Model file for the job. Use its own axes, mm. A direction names the side the tool comes from. Give positions to 0.01 mm unless a question says otherwise; leave off trailing zeros. Loops run counter-clockwise (first coordinate to the right, second up) from the corner with the lowest first, then second, coordinate; pieces in that order, holes last. Notation, with made-up numbers: M 49,34 L 54,34 A25 ccw 54,51 Z; hole C -3.5,14 d11. An arc over 180 degrees is marked long. Use CSV: the item, a comma, the result in double quotes. Start each with the question number.
(1) Flat gauge pins, fed straight in: P1, Ø1.1, axis at x = 0, y = -0.5, coming from the -Z side (3 decimals); P2, Ø0.8, axis at x = 0, z = -0.5, coming from the +Y side; P3, Ø1.4, axis at y = -1, z = 17.5, coming from the -X side (3 decimals). Where does each tip first touch, or does it go through?
(2) Tool access for faces 1 (the face through (0, -1.67, 17)), 2 (the face through (0, -1, -1.445)), 3 (the face through (0, -1, -1.245)), 4 (the face through (0, -1.47, 17)): list every direction of +Z, -Z, +X, -X, +Y, -Y with a clear straight run to the whole face (end or side of a thin tool).
(3) Wall check: line 1 along Z through (x, y) = (0, -1.4) (3 decimals); line 2 along Z through (x, y) = (0.35, -0.5) (3 decimals); line 3 along Y through (x, z) = (0.5, 12). Give the ranges that are in metal, low to high. Write a range as from..to.
(4) Slice it at A-A on y = -0.35. State how many separate pieces and enclosed holes the cut face has, and give its area (3 significant figures).
(5) Slice it at B-B on z = 10.25. List the corners of the cut face in (x, y).
```python
from build123d import *

# Parameters (mm, degrees)
SKETCH1_R        = 1.14
EXTRUSION1_DEPTH = 15.24
EXTRUSION2_DEPTH = 0.495
FILLET3_R        = 1.03


with BuildPart() as part:
    # Sketch1 → Extrusion1 (new body)
    with BuildSketch(Plane.XY):
        Circle(SKETCH1_R)
    extrude(amount=EXTRUSION1_DEPTH)

    # Sketch3 → Revolution3 (revolve, cut)
    with BuildSketch(Plane.YZ, mode=Mode.PRIVATE) as revolution3_sk:
        with BuildLine():
            Line((1.14, 12.96), (1.14, 14.1))
            ThreePointArc((1.14, 14.1), (1.101155442, 13.804946289), (0.98726896, 13.53))
            ThreePointArc((0.98726896, 13.53), (1.101155442, 13.255053711), (1.14, 12.96))
        make_face()
    revolution3 = revolve(revolution3_sk.sketch.rotate(Axis((0, 0, 14.1), (0, 0, -1)), 90), axis=Axis((0, 0, 14.1), (0, 0, -1)), mode=Mode.SUBTRACT)

    # Mirror2: Revolution3 across plane
    add(revolution3.mirror(Plane.XY.offset(7.62)), mode=Mode.SUBTRACT)

    # Sketch4 → Extrusion2 (add, symmetric)
    with BuildSketch(Plane.YZ):
        with BuildLine():
            Line((-0.1, 0), (0, 0))
            ThreePointArc((0, 0), (-0.050048254, 0.001099138), (-0.1, 0.004394435))
            Line((-0.1, 0.004394435), (-0.1, 0))
        make_face()
        with BuildLine():
            ThreePointArc((0, 0), (0.050048254, 0.001099138), (0.1, 0.004394435))
            Line((0.1, 0.004394435), (0.1, 0.138771336))
            Line((0.1, 0.138771336), (-0.1, 0.138771336))
            Line((-0.1, 0.138771336), (-0.1, 0.004394435))
            ThreePointArc((-0.1, 0.004394435), (-0.050048254, 0.001099138), (0, 0))
        make_face()
        Polygon((0.1, -1.445), (0.1, 0), (0, 0), (-0.1, 0), (-0.1, -1.245), (-1.67, -1.245), (-1.67, -2.925), (-1.47, -2.925), (-1.47, -1.445), align=None)
    extrusion2 = extrude(amount=EXTRUSION2_DEPTH, both=True)

    # Mirror3: Extrusion2 across plane
    add(extrusion2.mirror(Plane.XY.offset(7.62)))

    # Fillet3
    # the kernel refuses this fillet: 1.03 mm, written as the material it takes off along each edge
    with BuildSketch(Plane(origin=(0, 0, 15.24), x_dir=(1, 0, 0), z_dir=(0, -1, 0))) as fillet3_piece_1_section:
        with BuildLine():
            CenterArc((1.14 - FILLET3_R, -FILLET3_R), FILLET3_R, 0, 90)
            Line((1.14 - FILLET3_R, 0), (1.14, 0))
            Line((1.14, 0), (1.14, -FILLET3_R))
        make_face()
    fillet3_piece_1 = revolve(axis=Axis((0, 0, 15.24), (0, 0, 1)), mode=Mode.PRIVATE)
    fillet3_piece_1 = split(fillet3_piece_1, bisect_by=Plane(origin=(0.495, 4e-09, 15.000808078), z_dir=(1, 0, 0)), keep=Keep.TOP, mode=Mode.PRIVATE)
    add(fillet3_piece_1, mode=Mode.SUBTRACT)
    with BuildSketch(Plane(origin=(0, 0, 15.24), x_dir=(1, 0, 0), z_dir=(0, -1, 0))) as fillet3_piece_2_section:
        with BuildLine():
            CenterArc((1.14 - FILLET3_R, -FILLET3_R), FILLET3_R, 0, 90)
            Line((1.14 - FILLET3_R, 0), (1.14, 0))
            Line((1.14, 0), (1.14, -FILLET3_R))
        make_face()
    fillet3_piece_2 = revolve(axis=Axis((0, 0, 15.24), (0, 0, 1)), mode=Mode.PRIVATE)
    fillet3_piece_2 = split(fillet3_piece_2, bisect_by=Plane(origin=(0, 0.1, 15.013614208), z_dir=(0, 1, 0)), keep=Keep.TOP, mode=Mode.PRIVATE)
    add(fillet3_piece_2, mode=Mode.SUBTRACT)
    with BuildSketch(Plane(origin=(0, 0, 15.24), x_dir=(1, 0, 0), z_dir=(0, -1, 0))) as fillet3_piece_3_section:
        with BuildLine():
            CenterArc((1.14 - FILLET3_R, -FILLET3_R), FILLET3_R, 0, 90)
            Line((1.14 - FILLET3_R, 0), (1.14, 0))
            Line((1.14, 0), (1.14, -FILLET3_R))
        make_face()
    fillet3_piece_3 = revolve(axis=Axis((0, 0, 15.24), (0, 0, 1)), mode=Mode.PRIVATE)
    fillet3_piece_3 = split(fillet3_piece_3, bisect_by=Plane(origin=(8e-09, -0.1, 15.013614602), z_dir=(0, -1, 0)), keep=Keep.TOP, mode=Mode.PRIVATE)
    add(fillet3_piece_3, mode=Mode.SUBTRACT)
    with BuildSketch(Plane(origin=(0, 0, 15.24), x_dir=(1, 0, 0), z_dir=(0, -1, 0))) as fillet3_piece_4_section:
        with BuildLine():
            CenterArc((1.14 - FILLET3_R, -FILLET3_R), FILLET3_R, 0, 90)
            Line((1.14 - FILLET3_R, 0), (1.14, 0))
            Line((1.14, 0), (1.14, -FILLET3_R))
        make_face()
    fillet3_piece_4 = revolve(axis=Axis((0, 0, 15.24), (0, 0, 1)), mode=Mode.PRIVATE)
    fillet3_piece_4 = split(fillet3_piece_4, bisect_by=Plane(origin=(-0.495, -1e-09, 15.000807979), z_dir=(-1, 0, 0)), keep=Keep.TOP, mode=Mode.PRIVATE)
    add(fillet3_piece_4, mode=Mode.SUBTRACT)
    with BuildSketch(Plane(origin=(0, 0, 0), x_dir=(1, 0, 0), z_dir=(0, -1, 0))) as fillet3_piece_5_section:
        with BuildLine():
            CenterArc((1.14 - FILLET3_R, FILLET3_R), FILLET3_R, 270, 90)
            Line((1.14 - FILLET3_R, 0), (1.14, 0))
            Line((1.14, 0), (1.14, FILLET3_R))
        make_face()
    fillet3_piece_5 = revolve(axis=Axis((0, 0, 0), (0, 0, 1)), mode=Mode.PRIVATE)
    fillet3_piece_5 = split(fillet3_piece_5, bisect_by=Plane(origin=(0.495, 4e-09, 0.239191922), z_dir=(1, 0, 0)), keep=Keep.TOP, mode=Mode.PRIVATE)
    add(fillet3_piece_5, mode=Mode.SUBTRACT)
    with BuildSketch(Plane(origin=(0, 0, 0), x_dir=(1, 0, 0), z_dir=(0, -1, 0))) as fillet3_piece_6_section:
        with BuildLine():
            CenterArc((1.14 - FILLET3_R, FILLET3_R), FILLET3_R, 270, 90)
            Line((1.14 - FILLET3_R, 0), (1.14, 0))
            Line((1.14, 0), (1.14, FILLET3_R))
        make_face()
    fillet3_piece_6 = revolve(axis=Axis((0, 0, 0), (0, 0, 1)), mode=Mode.PRIVATE)
    fillet3_piece_6 = split(fillet3_piece_6, bisect_by=Plane(origin=(0, 0.1, 0.226385792), z_dir=(0, 1, 0)), keep=Keep.TOP, mode=Mode.PRIVATE)
    add(fillet3_piece_6, mode=Mode.SUBTRACT)
    with BuildSketch(Plane(origin=(0, 0, 0), x_dir=(1, 0, 0), z_dir=(0, -1, 0))) as fillet3_piece_7_section:
        with BuildLine():
            CenterArc((1.14 - FILLET3_R, FILLET3_R), FILLET3_R, 270, 90)
            Line((1.14 - FILLET3_R, 0), (1.14, 0))
            Line((1.14, 0), (1.14, FILLET3_R))
        make_face()
    fillet3_piece_7 = revolve(axis=Axis((0, 0, 0), (0, 0, 1)), mode=Mode.PRIVATE)
    fillet3_piece_7 = split(fillet3_piece_7, bisect_by=Plane(origin=(8e-09, -0.1, 0.226385398), z_dir=(0, -1, 0)), keep=Keep.TOP, mode=Mode.PRIVATE)
    add(fillet3_piece_7, mode=Mode.SUBTRACT)
    with BuildSketch(Plane(origin=(0, 0, 0), x_dir=(1, 0, 0), z_dir=(0, -1, 0))) as fillet3_piece_8_section:
        with BuildLine():
            CenterArc((1.14 - FILLET3_R, FILLET3_R), FILLET3_R, 270, 90)
            Line((1.14 - FILLET3_R, 0), (1.14, 0))
            Line((1.14, 0), (1.14, FILLET3_R))
        make_face()
    fillet3_piece_8 = revolve(axis=Axis((0, 0, 0), (0, 0, 1)), mode=Mode.PRIVATE)
    fillet3_piece_8 = split(fillet3_piece_8, bisect_by=Plane(origin=(-0.495, -1e-09, 0.239192021), z_dir=(-1, 0, 0)), keep=Keep.TOP, mode=Mode.PRIVATE)
    add(fillet3_piece_8, mode=Mode.SUBTRACT)


solid = part.part
```
Reply:
1,P1,"stops at z = -1.445"
1,P2,"stops at y = 0.1"
1,P3,"stops at x = -0.495"
2,face 1,"+Z, -Z, +X, -X, -Y"
2,face 2,"-Z, +X, -X, +Y"
2,face 3,"+X, -X, -Y"
2,face 4,"+Z, +X, -X, +Y"
3,line 1,"z = -1.445..-1.245, 16.485..16.685"
3,line 2,"z = -1.445..-1.245, 0.13..15.11, 16.485..16.685"
3,line 3,"y = -1.02..1.02"
4,separate pieces,"3"
4,enclosed holes,"0"
4,area,"32.2 mm^2"
5,outline,"C 0,0 d2.28"
